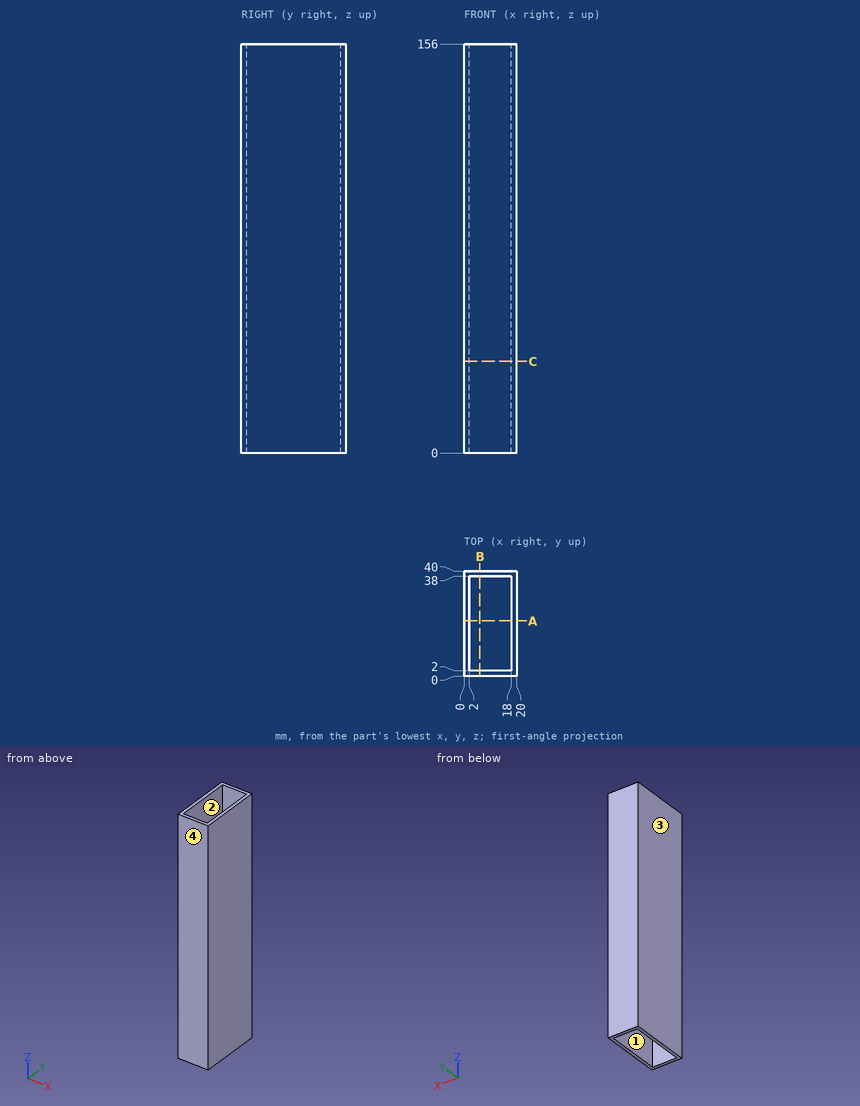
Verification items for this drawing (mm, ordinates from the low corner). Round coordinates to 2 decimals unless told otherwise and drop trailing zeros. Order: outer loops, then holes, each group sorted by start corner. A loop starts at its lowest first (then second) coordinate and runs counter-clockwise, first axis right, second up. Notation, with made-up numbers: (-24.75, 12) - (22.25, 12) arc R14 ccw to (22.25, 28) - close; hole circle Ø2 at (11, 31). An arc over 180 degrees is marked (long way). Use CSV: the item, a comma, the result in double quotes. Start each with the question number.
1) Section check A-A, the plane y = 21. Record the cut outline in (x, z).
2) Section check B-B, the plane x = 6. Record the cut outline in (y, z), plus the area to 3 significant figures.
3) Mould release check, pull along X, two halves, no side actions. Record for the marked faces 1, 2, 3 and 4: +X half, -X half, draft (parallel to the pull), parting line (faces both ways), or undercut.
4) Thickness scan on L1, parallel to X at y = 32, z = 110; L2, parallel to Y at x = 5, z = 135. Record the ranges inside material, lowest first.
5) Go/stop test with a flat-tipped pin: P1, Ø10, axis at x = 2.5, y = 12.5, coming from the -Z side. Record where the tip stops, or that it passes through.
6) Section check C-C, the plane z = 35. Record the cut outline in (x, y), plus the area to 3 significant figures.
Answers:
1,outline,"(0, 0) - (2, 0) - (2, 156) - (0, 156) - close; (18, 0) - (20, 0) - (20, 156) - (18, 156) - close"
2,outline,"(0, 0) - (2, 0) - (2, 156) - (0, 156) - close; (38, 0) - (40, 0) - (40, 156) - (38, 156) - close"
2,area,"624 mm²"
3,face 1,"undercut"
3,face 2,"undercut"
3,face 3,"-X half"
3,face 4,"draft"
4,L1,"x = 0 to 2, 18 to 20"
4,L2,"y = 0 to 2, 38 to 40"
5,P1,"stops at z = 0"
6,outline,"(0, 0) - (20, 0) - (20, 40) - (0, 40) - close; hole (2, 2) - (18, 2) - (18, 38) - (2, 38) - close"
6,area,"224 mm²"
